Input: dimensioned drawing with shaded views. Units: mm. Origin: part minimum x, y, z. A direction names the side the tool comes from. Coordinates: 2 decimals unless noted, no trailing zeros. Write each loop counter-clockwise with the first axis right and the second up, starting at its lowest first coordinate (ties: lowest second). Pieces come first, ordered by that corner, then holes. Notation, with made-up numbers: M 45,-36 L 53,-36 A22 cw 53,-23 Z; hole C 81,73.5 d6. An arc over 180 degrees is marked long. Use one line per item in the form item = value.
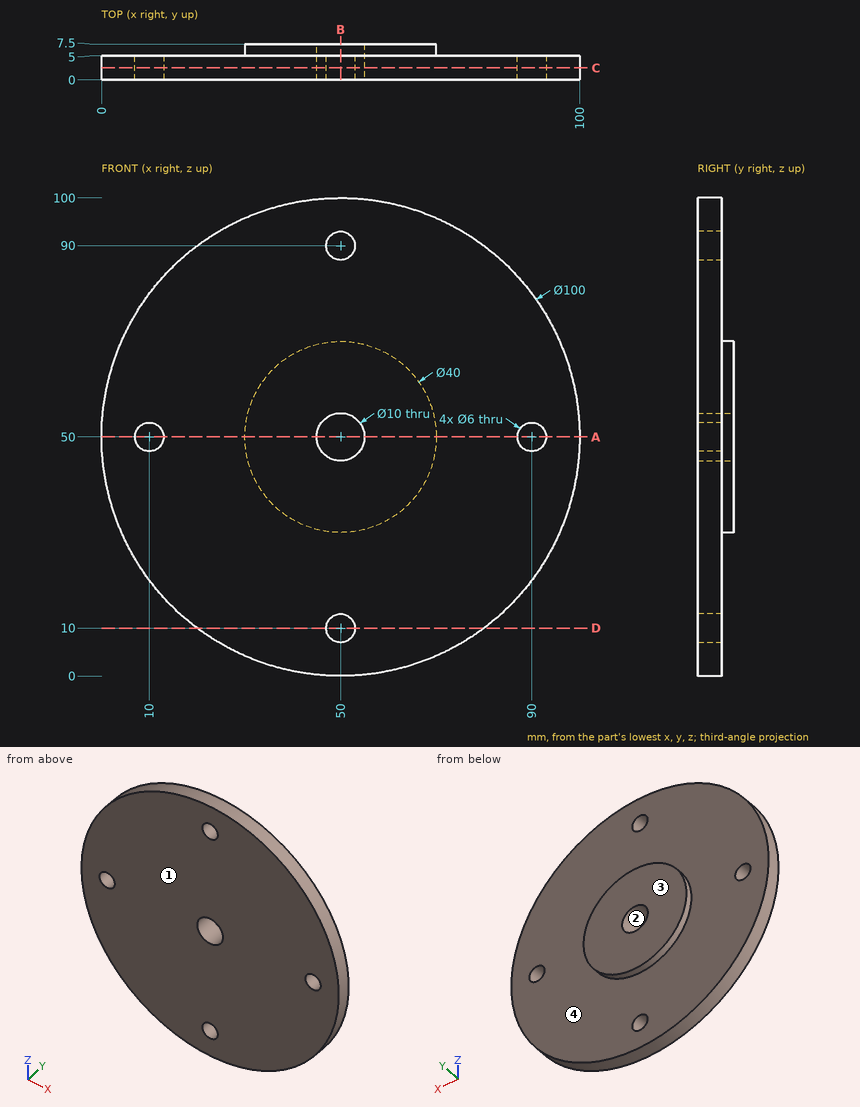
(1) Section query C-C on y = 2.5. Return the cut outline in (x, z).
Computed:
outline = C 50,50 d100; hole C 10,50 d6; hole C 50,50 d10; hole C 50,10 d6; hole C 50,90 d6; hole C 90,50 d6
(2) Pull-direction query (Z, two-part tool) for the marked faces 1 and 2; classes: pulls with the +Z half, pulls with the -Z half, needs draft (parallel to the pull), parting line crosses it, or undercut.
Computed:
face_1 = needs draft
face_2 = undercut
(3) Section query D-D on z = 10. Return the cut outline in (x, y).
Computed:
outline = M 20,0 L 47,0 L 47,5 L 20,5 Z; M 53,0 L 80,0 L 80,5 L 53,5 Z
(4) Section query B-B on x = 50. Return the cut outline in (y, z), plus the area to 3 significant figures.
Computed:
outline = M 0,0 L 5,0 L 5,7 L 0,7 Z; M 0,13 L 5,13 L 5,30 L 7.5,30 L 7.5,45 L 0,45 Z; M 0,55 L 7.5,55 L 7.5,70 L 5,70 L 5,87 L 0,87 Z; M 0,93 L 5,93 L 5,100 L 0,100 Z
area = 465 mm^2
(5) Line query: probe 1 along Z at (x, y) = (50, 1.8); probe 2 along Z at (x, y) = (50, 6.75); probe 3 along Y at (x, z) = (40, 72.5). Output: solid intervals per line, ascending.
Computed:
probe_1 = 0 to 7, 13 to 45, 55 to 87, 93 to 100
probe_2 = 30 to 45, 55 to 70
probe_3 = 0 to 5
(6) Section query A-A on z = 50. Return the cut outline in (x, y), plus the area to 3 significant figures.
Computed:
outline = M 0,0 L 7,0 L 7,5 L 0,5 Z; M 13,0 L 45,0 L 45,7.5 L 30,7.5 L 30,5 L 13,5 Z; M 55,0 L 87,0 L 87,5 L 70,5 L 70,7.5 L 55,7.5 Z; M 93,0 L 100,0 L 100,5 L 93,5 Z
area = 465 mm^2
(7) Set-up query: the marked faces 3 and 4. Return all of +Z, -Z, +X, -X, +Y, -Y with unobstructed straight access to the full face (end or side cutting, diameter ignored); none if empty.
Computed:
face_3 = +Z, -Z, +X, -X, +Y
face_4 = +Y
(8) First-contact query: pin 1 Ø3.5 at (x, z) = (50, 90) entering from -Y; pin 2 Ø7 at (x, z) = (10, 50) entering from +Y; pin 3 Ø1.5 at (x, y) = (41, 1) entering from +Z; pin 4 Ø4 at (y, z) = (3, 20.5) entering from +X. Flat tips, straight axial feed; report the tip coordinate or a pass-through.
Computed:
pin_1 = through
pin_2 = 5
pin_3 = 99.31
pin_4 = 91.76
